```python
from build123d import *

# Parameters (mm, degrees)
F1_W      = 127
F1_H      = 38.1
F2_DEPTH  = 3.175
F4_W      = 127
F4_H      = 3.175
F5_DEPTH  = 76.2
F7_W      = 12.7
F7_H      = 31.75
F8_DEPTH  = 12.7
F6_R      = 2.667
F9_DEPTH  = 25.4
F9_TAPER  = -2
F10_R     = 3.17499
F12_DEPTH = 6.35
F14_DEPTH = 6.35
F15_R     = 4.7625
F16_DEPTH = 6.35
F17_R     = 1.905
F18_DEPTH = 25.4
F19_SIZE  = 2.54
F20_SIZE  = 2.54
F21_SIZE  = 7.62


# Not quite as in the source:
# - a fillet or chamfer is up to 0.001 mm smaller than in the source, because OpenCascade refuses the exact size


with BuildPart() as f2:
    # F1 (on Top) → F2 (new body)
    with BuildSketch(Plane.XY):
        with Locations((63.5, -19.05)):
            Rectangle(F1_W, F1_H)
    extrude(amount=F2_DEPTH)

    # F4 (on face) → F5 (join)
    with BuildSketch(Plane.XY.offset(3.175)):
        with Locations((63.5, -1.5875)):
            Rectangle(F4_W, F4_H)
    extrude(amount=F5_DEPTH)

    # F7 (on Top) → F8 (join)
    with BuildSketch(Plane.XY):
        with Locations((38.1, -22.225)):
            Rectangle(F7_W, F7_H)
        with Locations((101.6, -22.3082778975)):
            Rectangle(F7_W, F7_H)
    extrude(amount=F8_DEPTH)

    # F6 (on Top) → F9 (cut)
    with BuildSketch(Plane.XY):
        with Locations((38.1, -22.225)):
            Circle(F6_R)
        with Locations((101.6, -22.225)):
            Circle(F6_R)
    extrude(amount=F9_DEPTH, taper=F9_TAPER, mode=Mode.SUBTRACT)

    # F10 (radius 3.175 in the source; OpenCascade refuses exactly that, so slightly less here)
    f10_edges = [f2.edges().sort_by_distance(p)[0] for p in [
        (0, -19.05, 0),
        (127, -19.05, 0),
    ]]
    fillet(f10_edges, radius=F10_R)

    # F11 (on face) → F12 (join)
    with BuildSketch(Plane(origin=(0, 0, 0), x_dir=(0, -1, 0), z_dir=(-1, 0, 0))):
        Polygon((32.4499383569, 3.175), (0, 22.225), (0, 3.175), align=None)
    extrude(amount=-F12_DEPTH)

    # F13 (on face) → F14 (join)
    with BuildSketch(Plane.YZ.offset(127)):
        Polygon((0, 3.175), (0, 20.8942663938), (-31.75, 3.175), align=None)
    extrude(amount=-F14_DEPTH)

    # F15 (on face) → F16 (join)
    with BuildSketch(Plane.XZ.offset(3.175)):
        with Locations((19.05, 60.3252180792)):
            Circle(F15_R)
        with Locations((47.8610846677, 55.9717772163)):
            Circle(F15_R)
        with Locations((76.4872658529, 60.3252180792)):
            Circle(F15_R)
        with Locations((107.9343466558, 57.469660566)):
            Circle(F15_R)
        with Locations((19.0343466558, 31.75)):
            Circle(F15_R)
        with Locations((69.0070766487, 31.75)):
            Circle(F15_R)
        with Locations((114.2843466558, 31.75)):
            Circle(F15_R)
    extrude(amount=F16_DEPTH)

    # F17 (on Front) → F18 (cut)
    with BuildSketch(Plane.XZ):
        with Locations((19.05, 60.325)):
            Circle(F17_R)
        with Locations((47.8767380118, 55.9715591371)):
            Circle(F17_R)
        with Locations((76.5029191971, 60.325)):
            Circle(F17_R)
        with Locations((107.95, 57.4694424868)):
            Circle(F17_R)
        with Locations((19.05, 31.75)):
            Circle(F17_R)
        with Locations((69.0227299929, 31.75)):
            Circle(F17_R)
        with Locations((114.3, 31.75)):
            Circle(F17_R)
    extrude(amount=F18_DEPTH, mode=Mode.SUBTRACT)

    # F19
    f19_edges = [f2.edges().sort_by_distance(p)[0] for p in [
        (17.145, -9.525, 60.325),
        (45.971738, -9.525, 55.971559),
        (74.597919, -9.525, 60.325),
        (17.145, -9.525, 31.75),
        (106.045, -9.525, 57.469442),
        (112.395, -9.525, 31.75),
        (67.11773, -9.525, 31.75),
    ]]
    chamfer(f19_edges, length=F19_SIZE)

    # F20
    f20_edges = [f2.edges().sort_by_distance(p)[0] for p in [
        (63.5, -3.175, 79.375),
    ]]
    chamfer(f20_edges, length=F20_SIZE)

    # F21
    f21_edges = [f2.edges().sort_by_distance(p)[0] for p in [
        (38.1, -38.1, 12.7),
        (101.6, -38.183278, 12.7),
    ]]
    chamfer(f21_edges, length=F21_SIZE)


solid = f2.part
```
Geometry check sheet. Reference: the model listing, model coordinates, mm. A direction names the side the tool comes from. Give positions to 0.01 mm unless a question says otherwise; leave off trailing zeros. Order: outer loops, then holes, each group sorted by start corner. A loop starts at its lowest first (then second) coordinate and runs counter-clockwise, first axis right, second up.
1. Thickness scan on L1, parallel to Z at x = 107.95, y = -4 (3 decimals); L2, parallel to X at y = -3.5, z = 30; L3, parallel to Z at x = 107, y = -4 (3 decimals). Record the ranges inside material, lowest first.
2. Section check C-C, the plane x = 114.3. Enter the section's corners in (y, z) (3 decimals).
3. Gauge pin test, flat ends, axial feed: pin 1 Ø1 at (x, z) = (117, 2) entering from -Y; pin 2 Ø1 at (x, z) = (82.5, 51.5) entering from +Y; pin 3 Ø3 at (x, z) = (116, 32) entering from -Y; pin 4 Ø7.5 at (x, z) = (18, 32.5) entering from -Y (3 decimals). Record the tip position at first contact, or that the pin passes through.
4. Section check A-A, the plane z = 31.75. Give the number of separate pieces and of enclosed holes in the cut face, and give its area (3 significant figures).
5. Section check D-D, the plane x = 61.5. Enter the section's corners in (y, z) (3 decimals).
6. Release check for a two-part mould opening along Z. For faces 4 (the face through (0.95, -18.78, 0.91)), 5 (the face through (70.9, -7.1, 32.5)), 6 (the face through (47, -38.1, 2)) record: pulls with the +Z half, pulls with the -Z half, needs draft (parallel to the pull), parting line crosses it, or undercut.
7. Access from +Z, -Z, +X, -X, +Y, -Y to the whole of each face (thin tool, end or side, straight path). Record for faces 1 (the face through (64, 0, 39)), 2 (the face through (120.65, -11, 8)), 3 (the face through (15.524, -6.306, 34.969)).
Values follow:
1. L1: z = 0 to 3.175, 52.707 to 55.564, 59.374 to 62.232
1. L2: x = 14.61 to 18.3, 19.8 to 23.46, 64.58 to 68.27, 69.78 to 73.44, 109.86 to 113.55, 115.05 to 118.71
1. L3: z = 0 to 3.175, 52.8 to 55.818, 59.121 to 62.14
2. outline: (-38.1, 0) - (0, 0) - (0, 29.845) - (-6.985, 29.845) - (-9.525, 27.305) - (-9.525, 26.988) - (-3.175, 26.988) - (-3.175, 3.175) - (-38.1, 3.175) - close; (-9.525, 36.195) - (-6.985, 33.655) - (0, 33.655) - (0, 79.375) - (-0.635, 79.375) - (-3.175, 76.835) - (-3.175, 36.512) - (-9.525, 36.512) - close
3. pin 1: stops at y = -38.1
3. pin 2: stops at y = 0
3. pin 3: stops at y = -8.3
3. pin 4: stops at y = -9.525
4. separate pieces: 4
4. enclosed holes: 0
4. area: 456 mm2
5. outline: (-38.1, 0) - (0, 0) - (0, 79.375) - (-0.635, 79.375) - (-3.175, 76.835) - (-3.175, 3.175) - (-38.1, 3.175) - close
6. face 4: pulls with the -Z half
6. face 5: undercut
6. face 6: needs draft
7. face 1: +Z, -Z, +X, -X, +Y
7. face 2: +Z, -Y
7. face 3: -Y
